Here's how the part is built. I have some questions about the finished solid (model axes, mm). Face numbers are marked on the shaded views. A direction names the side the tool comes from. Round coordinates to 2 decimals unless told otherwise and drop trailing zeros. Write each loop counter-clockwise with the first axis right and the second up, starting at its lowest first coordinate (ties: lowest second). Pieces come first, ordered by that corner, then holes. Notation, with made-up numbers: (41.5, 70.25) - (78.5, 70.25) arc R12 ccw to (78.5, 87.25) - close; hole circle Ø4 at (6.25, 29.25). An arc over 180 degrees is marked (long way). Use one line per item in the form item = value. Start each with the question number.
1. I want a section at B-B, the plane z = 8. List the corners of the cut face in (x, y) for me (3 decimals).
2. Will these pins go through, and if not, where does the flat tip stop? pin 1 (2 mm diameter, centred on x = 2.5, y = 1.5, fed in from -Z); pin 2 (3 mm diameter, centred on x = -4.5, y = -2.5, fed in from +Z); pin 3 (3 mm diameter, centred on x = 4, y = -0.5, fed in from +Z).
3. I want a section at A-A, the plane z = 7. List the corners of the cut face in (x, y) for me (3 decimals).
4. I want a section at C-C, the plane x = -1.25. List the corners of the cut face in (y, z) for me (3 decimals).
5. If I drill on line 1 along X through (y, z) = (2, 7.75); line 2 along X through (y, z) = (-2.5, 8.5); line 3 along Z through (x, y) = (-8.25, 0.25), over which ranges is the centre line in solid material (lowest first)?
6. Which directions (+Z, -Z, +X, -X, +Y, -Y) give clear straight access to the entire face, cutting with the end or side of a thin tool? Please do the marked faces 1 and 2.
7. We'd pull the mould along X, two halves only. Please class the marked faces 3, 4 and 5: +X half, -X half, draft (parallel to the pull), parting line (faces both ways), or undercut.
```python
from build123d import *

# Parameters (mm, degrees)
BOSS_EXTRUDE1_DEPTH     = 3.175
CUT_EXTRUDE1_DEPTH      = 14.942762459
CUT_EXTRUDE1_DEPTH_BACK = 14.942762459


with BuildPart() as part:
    # Sketch1 → Boss-Extrude1 (new, symmetric)
    with BuildSketch(Plane(origin=(0, 0, 0), x_dir=(1, 0, 0), z_dir=(0, 1, 0))):
        with BuildLine():
            Line((0.050388708, -9.493548387), (2.317880549, -8.903225806))
            ThreePointArc((2.317880549, -8.903225806), (7.278890748, -5.62652197), (9.2, 0))
            Line((9.2, 0), (9.3, 0))
            ThreePointArc((9.3, 0), (7.358009126, -5.687679817), (2.343074903, -9))
            Line((2.343074903, -9), (0.063226066, -9.593539621))
            ThreePointArc((0.063226066, -9.593539621), (0.03837284, -9.598354384), (0.013110494, -9.599991048))
            ThreePointArc((0.013110494, -9.599991048), (-6.783588256, -6.792858777), (-9.6, 0))
            Line((-9.6, 0), (-9.5, 0))
            ThreePointArc((-9.5, 0), (-6.717514421, -6.717514421), (0, -9.5))
            ThreePointArc((0, -9.5), (0.025400025, -9.49838054), (0.050388708, -9.493548387))
        make_face()
    extrude(amount=BOSS_EXTRUDE1_DEPTH, both=True)

    # Sketch2 → Cut-Extrude1 (cut, two sides: drawn at the far end of the back side and taken through both)
    with BuildSketch(Plane(origin=(0, 0, 0), x_dir=(0, 0, -1), z_dir=(1, 0, 0)).offset(-CUT_EXTRUDE1_DEPTH_BACK)):
        Polygon((0, 3.55), (0, 2.8), (-0.649519053, 3.175), align=None)
        Polygon((0, 2.8), (0, 2.05), (-0.649519053, 2.425), align=None)
        Polygon((0, 2.05), (0, 1.3), (-0.649519053, 1.675), align=None)
        Polygon((0, 1.3), (0, 0.55), (-0.649519053, 0.925), align=None)
        Polygon((0, 0.55), (0, -0.2), (-0.649519053, 0.175), align=None)
        Polygon((0, -0.2), (0, -0.95), (-0.649519053, -0.575), align=None)
        Polygon((0, -0.95), (0, -1.7), (-0.649519053, -1.325), align=None)
        Polygon((0, -1.7), (0, -2.45), (-0.649519053, -2.075), align=None)
        Polygon((0, -2.45), (0, -3.2), (-0.649519053, -2.825), align=None)
    extrude(amount=CUT_EXTRUDE1_DEPTH + CUT_EXTRUDE1_DEPTH_BACK, mode=Mode.SUBTRACT)


solid = part.part
```
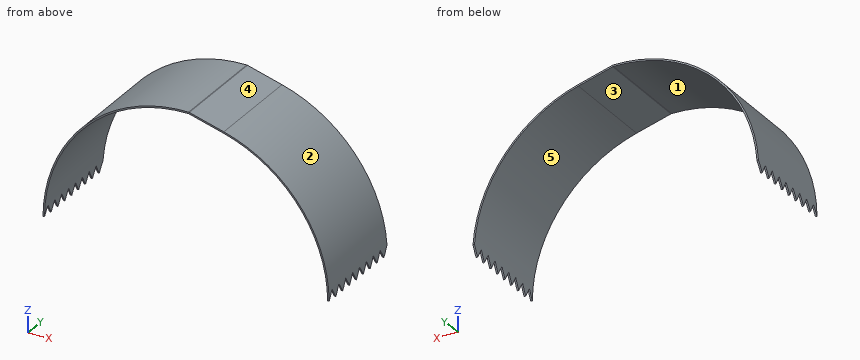
Model answer:
q1.outline = (-5.307, -3.175) - (-5.123, -3.175) - (-5.123, 3.175) - (-5.307, 3.175) - close; (4.543, -3.175) - (4.742, -3.175) - (4.742, 3.175) - (4.543, 3.175) - close
q2.pin_1 = 8.51
q2.pin_2 = 9.12
q2.pin_3 = 8.96
q3.outline = (-6.57, -3.175) - (-6.423, -3.175) - (-6.423, 3.175) - (-6.57, 3.175) - close; (5.97, -3.175) - (6.123, -3.175) - (6.123, 3.175) - (5.97, 3.175) - close
q4.outline = (-3.175, 9.417) - (3.175, 9.417) - (3.175, 9.518) - (-3.175, 9.518) - close
q5.line_1 = -5.67 to -5.49, 4.96 to 5.14
q5.line_2 = -4.46 to -4.24, 3.52 to 3.77
q5.line_3 = 4.71 to 4.91
q6.face_1 = -Z, +Y, -Y
q6.face_2 = +Z, +X, +Y, -Y
q7.face_3 = undercut
q7.face_4 = +X half
q7.face_5 = undercut
